Design review of the part built by this model. Coordinates are the model's own, in mm. A direction names the side the tool comes from. Round coordinates to 2 decimals unless told otherwise and drop trailing zeros. Write each loop counter-clockwise with the first axis right and the second up, starting at its lowest first coordinate (ties: lowest second). Pieces come first, ordered by that corner, then holes. Notation, with made-up numbers: M 9.5,56 L 46.5,56 A28 ccw 46.5,75 Z; hole C 68,63 d1. An arc over 180 degrees is marked long. Use CSV: the item, a comma, the result in double quotes.
from build123d import *

# Parameters (mm, degrees)
SKETCH_W     = 260
SKETCH_H     = 450
PAD_DEPTH    = 18
SKETCH001_W  = 60
SKETCH001_H  = 18
POCKET_DEPTH = 12
CHAMFER_SIZE = 15
FILLET_R     = 10


with BuildPart() as part:
    # Sketch → Pad (new body)
    with BuildSketch(Plane.XY):
        Rectangle(SKETCH_W, SKETCH_H)
    extrude(amount=PAD_DEPTH)

    # Sketch001 → Pocket (cut)
    with BuildSketch(Plane.XY.offset(18)):
        with Locations((0, 151)):
            Rectangle(SKETCH001_W, SKETCH001_H)
    pocket = extrude(amount=-POCKET_DEPTH, mode=Mode.SUBTRACT)

    # Mirrored: Pocket across Sketch001 H_Axis
    add(pocket.mirror(Plane(origin=(0, 0, 18), x_dir=(0, 0, 1), z_dir=(0, 1, 0))), mode=Mode.SUBTRACT)

    # Chamfer
    chamfer_edges = [part.edges().sort_by_distance(p)[0] for p in [
        (-130, -225, 9),
        (-130, 225, 9),
        (130, 225, 9),
        (130, -225, 9),
    ]]
    chamfer(chamfer_edges, length=CHAMFER_SIZE)

    # Fillet
    fillet_edges = [part.edges().sort_by_distance(p)[0] for p in [
        (115, -225, 9),
        (130, -210, 9),
        (-115, -225, 9),
        (-130, -210, 9),
        (-130, 210, 9),
        (-115, 225, 9),
        (115, 225, 9),
        (130, 210, 9),
    ]]
    fillet(fillet_edges, radius=FILLET_R)


solid = part.part
1) Machinability: for faces 4 (the face through (-130, -3, 9)), 5 (the face through (-30, 151, 12)), which of the approach directions +Z, -Z, +X, -X, +Y, -Y give a long, thin tool a straight path to every point of the face, cutting with its end or side? Answer none if there is none.
Answers:
face 4,"+Z, -Z, -X, +Y, -Y"
face 5,"+Z"
2) Add section B-B on z = 10. Write out the cut boundary in (x, y), then the cut area to 3 significant figures.
Answers:
outline,"M -130,-205.86 A10 ccw -127.07,-212.93 L -117.93,-222.07 A10 ccw -110.86,-225 L 110.86,-225 A10 ccw 117.93,-222.07 L 127.07,-212.93 A10 ccw 130,-205.86 L 130,205.86 A10 ccw 127.07,212.93 L 117.93,222.07 A10 ccw 110.86,225 L -110.86,225 A10 ccw -117.93,222.07 L -127.07,212.93 A10 ccw -130,205.86 Z; hole M -30,-160 L 30,-160 L 30,-142 L -30,-142 Z; hole M -30,142 L 30,142 L 30,160 L -30,160 Z"
area,"114,000 mm²"
3) Wall thickness on line 1 along Y through (x, z) = (1, 7.25); line 2 along Y through (x, z) = (-118, 1); line 3 along Y through (x, z) = (-112.5, 3.5): over which ranges is each line inside the solid? List them lowest first. Write a range as [from, to].
Answers:
line 1,"[-225, -160], [-142, 142], [160, 225]"
line 2,"[-222, 222]"
line 3,"[-224.86, 224.86]"
4) Add section A-A on x = 1. Write out the cut boundary in (y, z).
Answers:
outline,"M -225,0 L 225,0 L 225,18 L 160,18 L 160,6 L 142,6 L 142,18 L -142,18 L -142,6 L -160,6 L -160,18 L -225,18 Z"
5) The part is to be moulded in two halves that separate along X. For faces 1 (the face through (130, -3, 9)), 2 (the face through (0, -142, 12)), 3 (the face through (-2, -225, 9)), say which applies: released by +X, released by -X, zero draft, split by the parting line, or undercut.
Answers:
face 1,"released by +X"
face 2,"undercut"
face 3,"zero draft"
